```python
from build123d import *

# Parameters (mm, degrees)
SKETCH2_R               = 28.575
SKETCH2_R_2             = 14.2875
BOSS_EXTRUDE1_DEPTH     = 19.05
BOSS_EXTRUDE3_DEPTH     = 6.35
CUT_EXTRUDE3_DEPTH      = 105.251956428
CUT_EXTRUDE3_DEPTH_BACK = 105.251956428
SKETCH6_R               = 6.35
SKETCH6_W               = 3.341744035
SKETCH6_H               = 6.35


with BuildPart() as part:
    # Sketch2 → Boss-Extrude1 (new, symmetric)
    with BuildSketch(Plane.XY):
        with Locations(Location((-0.0317959, 0.136414209, 0), (0, 0, 180))):
            Circle(SKETCH2_R)
        with Locations(Location((-0.0317959, 0.136414209, 0), (0, 0, 180))):
            Circle(SKETCH2_R_2, mode=Mode.SUBTRACT)
    extrude(amount=BOSS_EXTRUDE1_DEPTH, both=True)

    # Sketch5 → Boss-Extrude3 (add, symmetric)
    with BuildSketch(Plane.XY):
        with BuildLine():
            Line((4.364357946, 28.371223512), (84.960511793, 15.822419377))
            ThreePointArc((84.960511793, 15.822419377), (98.3932041, 0.136414209), (84.960511793, -15.549590959))
            Line((84.960511793, -15.549590959), (4.364357946, -28.098395094))
            ThreePointArc((4.364357946, -28.098395094), (28.5432041, 0.136414209), (4.364357946, 28.371223512))
        make_face()
    extrude(amount=BOSS_EXTRUDE3_DEPTH, both=True)

    # Sketch6 → Cut-Extrude3 (cut, two sides: drawn at the far end of the back side and taken through both)
    with BuildSketch(Plane.XY.offset(-CUT_EXTRUDE3_DEPTH_BACK)):
        with Locations((82.5182041, 0.136414209)):
            Circle(SKETCH6_R)
        with Locations((15.569332083, 0.136414209)):
            Rectangle(SKETCH6_W, SKETCH6_H)
    extrude(amount=CUT_EXTRUDE3_DEPTH + CUT_EXTRUDE3_DEPTH_BACK, mode=Mode.SUBTRACT)


solid = part.part
```
Input: part model. Units: mm. Frame: model coordinates. A direction names the side the tool comes from. Give positions to 0.01 mm unless a question says otherwise; leave off trailing zeros. Order: outer loops, then holes, each group sorted by start corner. A loop starts at its lowest first (then second) coordinate and runs counter-clockwise, first axis right, second up. Notation, with made-up numbers: (-36.75, -39) -> (-11.75, -39) arc R21 cw to (-11.75, -20) -> close; hole circle Ø10 at (74, 2.25). An arc over 180 degrees is marked (long way). Write each question's results on one line, items separated by ' | '. Start each with the question number.
Item 1: Contact query for flat-ended pins moving along their axis: P1, Ø2, axis at y = -1.5, z = -7.5, coming from the -X side; P2, Ø6, axis at x = 28.5, y = 17, coming from the -Z side; P3, Ø6, axis at y = -18, z = -3, coming from the -X side. Output: stop coordinate, or through.
Item 2: Cut plane C-C on z = -2.5. Give the number of separate pieces and of enclosed holes in the cut face, then the cut area to 3 significant figures.
Item 3: Line query: line 1 (X direction, y = 0.5, z = -3.5); line 2 (X direction, y = -1, z = 1.5); line 3 (Z direction, x = 63.5, y = -13). Output: solid intervals per line, ascending.
Item 4: Cut plane B-B on y = 11. Return the cut outline in (x, z), then the cut area to 3 significant figures.
Item 5: Set-up query: faces 1 (the cylindrical face through (-27.3, -8.4, 0.3)), 2 (the flat face through (7, -13, -19.05)), 3 (the flat face through (16, -3.039, 0)). Return all of +Z, -Z, +X, -X, +Y, -Y with unobstructed straight access to the full face (end or side cutting, diameter ignored); none if empty.
Item 6: Cut plane A-A on x = -3.5. Return the cut outline in (y, z), then the cut area to 3 significant figures.
Item 7: Mould query, pull axis Y, two halves, no side actions, for faces 4 (the flat face through (45.227, -21.736, 0.089)), 5 (the flat face through (16, 3.311, 0)), 6 (the flat face through (7, -13, 19.05)). Classes: pulls with the +Y half, pulls with the -Y half, needs draft (parallel to the pull), parting line crosses it, or undercut.
Established:
1) P1: x = -28.6 | P2: z = -6.35 | P3: x = -24.27
2) separate pieces: 1 | enclosed holes: 2 | area: 4,600 mm^2
3) line 1: -28.6 to -14.31, 17.24 to 76.18, 88.86 to 98.39 | line 2: -28.58 to -14.27, 17.24 to 76.27, 88.77 to 98.35 | line 3: -6.35 to 6.35
4) outline: (-26.46, -19.05) -> (-9.31, -19.05) -> (-9.31, 19.05) -> (-26.46, 19.05) -> close; (9.25, -19.05) -> (26.4, -19.05) -> (26.4, -6.35) -> (94.09, -6.35) -> (94.09, 6.35) -> (26.4, 6.35) -> (26.4, 19.05) -> (9.25, 19.05) -> close | area: 2,170 mm^2
5) face 1: none | face 2: -Z, +X, -X, +Y, -Y | face 3: +Z, -Z
6) outline: (-28.23, -19.05) -> (-13.72, -19.05) -> (-13.72, 19.05) -> (-28.23, 19.05) -> close; (14, -19.05) -> (28.5, -19.05) -> (28.5, 19.05) -> (14, 19.05) -> close | area: 1,110 mm^2
7) face 4: pulls with the -Y half | face 5: undercut | face 6: needs draft
